Here's how the part is built. I have some questions about the finished solid (model axes, mm). A direction names the side the tool comes from. Coordinates: 2 decimals unless noted, no trailing zeros. Write each loop counter-clockwise with the first axis right and the second up, starting at its lowest first coordinate (ties: lowest second). Pieces come first, ordered by that corner, then holes.
Item 1: For faces 1 (the face through (96.517, -65.958, 3.944)), 2 (the face through (11.474, -33.344, 3.944)), 3 (the face through (96.154, -34.118, 3.944)), 4 (the face through (11.838, -65.184, 3.944)), which set-ups out of +Z, -Z, +X, -X, +Y, -Y let a thin tool reach every point of the face, with its end or its side?
Item 2: If I drill on line 1 (Z direction, x = 68, y = -55); line 2 (Y direction, x = 69, z = 19); line 3 (Y direction, x = 12.5, z = 17.5), over which ranges is the centre line in solid material (lowest first)?
Item 3: If we section it at A-A (z = 5.75): Please give me the cut outline in (x, y).
Item 4: If we section it at C-C (x = 26): Please give me the cut outline in (y, z), then the cut area to 3 significant figures.
Item 5: I'm going to push flat-ended pins straight in: pin 1 Ø12 at (x, y) = (74.5, -59.5) entering from +Z; pin 2 Ø6.5 at (x, y) = (9, -30.5) entering from +Z. Where does each tip first touch, or does it pass through?
Item 6: We'd pull the mould along Y, two halves only. Please class faces 5 (the face through (11.838, -34.118, 15.07)), 6 (the face through (100.9, -33.8, 9)), 7 (the face through (96.8, -70.4, 8)), 8 (the face through (18.71, -60.6, 19.01)): +Y half, -Y half, draft (parallel to the pull), parting line (faces both ways), or undercut.
Item 7: If we section it at B-B (y = -48.5): Please give me the cut outline in (x, z).
Item 8: If we section it at D-D (y = -61.5): Please give me the cut outline in (x, z), then the cut area to 3 significant figures.
from build123d import *

# Parameters (mm, degrees)
SKETCH002_W     = 98
SKETCH002_H     = 44
PAD001_DEPTH    = 20
POCKET001_DEPTH = 10
POCKET002_DEPTH = 8
SKETCH005_R     = 3
HOLE_DEPTH      = 25
SKETCH006_R     = 18
POCKET003_DEPTH = 2


with BuildPart() as part:
    # Sketch002 → Pad001 (new body)
    with BuildSketch(Plane.XY):
        with Locations((49, 22)):
            Rectangle(SKETCH002_W, SKETCH002_H)
    extrude(amount=PAD001_DEPTH)

    # Sketch003 (on Face6 of Pad001) → Pocket001 (cut)
    with BuildSketch(Plane.XY.offset(20)):
        with BuildLine():
            Line((0, 44), (0, 36))
            ThreePointArc((0, 36), (6.922499, 37.596876), (10, 44))
            Line((0, 44), (10, 44))
        make_face()
        with BuildLine():
            Line((0, 0), (0, 8))
            ThreePointArc((10, 0), (6.403124, 5.753905), (0, 8))
            Line((0, 0), (10, 0))
        make_face()
        with BuildLine():
            Line((98, 36), (98, 44))
            Line((98, 44), (88, 44))
            ThreePointArc((88, 44), (91.596876, 38.246095), (98, 36))
        make_face()
        with BuildLine():
            Line((88, 0), (98, 0))
            Line((98, 0), (98, 8))
            ThreePointArc((98, 8), (91.077501, 6.403124), (88, 0))
        make_face()
    extrude(amount=-POCKET001_DEPTH, mode=Mode.SUBTRACT)

    # Sketch004 (on Face2 of Pocket001) → Pocket002 (cut)
    with BuildSketch(Plane(origin=(0, 0, 0), x_dir=(1, 0, 0), z_dir=(0, 0, -1))):
        with BuildLine():
            Line((10, -44), (0, -44))
            Line((0, -36), (0, -44))
            ThreePointArc((10, -44), (6.403124, -38.246095), (0, -36))
        make_face()
        with BuildLine():
            Line((0, 0), (0, -8))
            ThreePointArc((0, -8), (6.922499, -6.403124), (10, 0))
            Line((0, 0), (10, 0))
        make_face()
        with BuildLine():
            Line((98, 0), (88, 0))
            ThreePointArc((88, 0), (91.596876, -5.753905), (98, -8))
            Line((98, 0), (98, -8))
        make_face()
        with BuildLine():
            Line((88, -44), (98, -44))
            Line((98, -44), (98, -36))
            ThreePointArc((98, -36), (91.077501, -37.596876), (88, -44))
        make_face()
    extrude(amount=-POCKET002_DEPTH, mode=Mode.SUBTRACT)

    # Sketch005 (on Face21 of Pocket002) → Hole (cut)
    with BuildSketch(Plane.XY.offset(10)):
        with Locations((3.5, 3.5)):
            Circle(SKETCH005_R)
        with Locations((3.5, 40.5)):
            Circle(SKETCH005_R)
        with Locations((94.5, 40.5)):
            Circle(SKETCH005_R)
        with Locations((94.5, 3.5)):
            Circle(SKETCH005_R)
    extrude(amount=-HOLE_DEPTH, mode=Mode.SUBTRACT)

    # Sketch006 (on Face8 of Hole) → Pocket003 (cut)
    with BuildSketch(Plane.XY.offset(20)):
        with Locations((28, 22)):
            Circle(SKETCH006_R)
        with Locations((70, 22)):
            Circle(SKETCH006_R)
    extrude(amount=-POCKET003_DEPTH, mode=Mode.SUBTRACT)


with BuildPart() as part_1:
    # Body001 placement: moved
    add(part.part.moved(Location((4.995761, -71.651041, 0))))


solid = part_1.part
Answer list:
1. face 1: -Z, +X, -Y
1. face 2: -Z, -X, +Y
1. face 3: -Z, +Y
1. face 4: -Z, -Y
2. line 1: z = 0 to 18
2. line 2: y = -71.65 to -66.62, -32.68 to -27.65
2. line 3: y = -66.92 to -33.54
3. outline: (5, -63.65) arc R8.2 cw to (15, -71.65) - (93, -71.65) arc R10.25 cw to (103, -63.65) - (103, -35.65) arc R8.2 cw to (93, -27.65) - (15, -27.65) arc R10.25 cw to (5, -35.65) - close
4. outline: (-71.65, 0) - (-27.65, 0) - (-27.65, 20) - (-33.07, 20) - (-33.07, 18) - (-66.24, 18) - (-66.24, 20) - (-71.65, 20) - close
4. area: 814 mm2
5. pin 1: stops at z = 18
5. pin 2: stops at z = 10
6. face 5: +Y half
6. face 6: undercut
6. face 7: draft
6. face 8: undercut
7. outline: (5, 0) - (103, 0) - (103, 20) - (92.96, 20) - (92.96, 18) - (57.03, 18) - (57.03, 20) - (50.96, 20) - (50.96, 18) - (15.03, 18) - (15.03, 20) - (5, 20) - close
8. outline: (5, 0) - (103, 0) - (103, 20) - (88.55, 20) - (88.55, 18) - (61.45, 18) - (61.45, 20) - (46.55, 20) - (46.55, 18) - (19.45, 18) - (19.45, 20) - (5, 20) - close
8. area: 1,850 mm2
